Part model, mm, in its own coordinate system. A direction names the side the tool comes from. Give positions to 0.01 mm unless a question says otherwise; leave off trailing zeros. Order: outer loops, then holes, each group sorted by start corner. A loop starts at its lowest first (then second) coordinate and runs counter-clockwise, first axis right, second up. Notation, with made-up numbers: M 87,-10 L 104,-10 A27 ccw 104,24 Z; hole C -1,49 d8. An arc over 180 degrees is marked long. Write each question's results on one line, items separated by ' | '. Start each with the question number.
from build123d import *

# Parameters (mm, degrees)
SKETCH_1_W                  = 55
SKETCH_1_H                  = 160
EXTRUDE_1_DEPTH             = 3
EXTRUDE_2_DEPTH             = 35
EXTRUDE_2_DEPTH_BACK        = 195
SKETCH_2_W                  = 35
SKETCH_2_H                  = 3
EXTRUDE_3_DEPTH             = 3
EXTRUDE_3_DEPTH_BACK        = 233
SKETCH_3_W                  = 15
SKETCH_3_H                  = 3
CUT_EXTRUDE_1_DEPTH         = 3
CUT_EXTRUDE_2_DEPTH         = 3
SKETCH_6_W                  = 77
SKETCH_6_H                  = 3
CUT_EXTRUDE_3_DEPTH         = 17
SKETCH_8_R                  = 2
CUT_EXTRUDE_4_DEPTH         = 3
SKETCH_9_W                  = 13
SKETCH_9_H                  = 20
CUT_EXTRUDE_5_DEPTH         = 3
FILLET_1_R                  = 10
SKETCH_10_R                 = 2
CUT_EXTRUDE_6_DEPTH         = 10
PATTERN_LINEAR_1_COUNT      = 4
PATTERN_LINEAR_1_PITCH      = 9
PATTERN_LINEAR_1_COUNT_DIR2 = 3
PATTERN_LINEAR_1_PITCH_DIR2 = 9
SKETCH_11_R                 = 2
CUT_EXTRUDE_7_DEPTH         = 10
PATTERN_LINEAR_2_COUNT      = 5
PATTERN_LINEAR_2_PITCH      = 9
PATTERN_LINEAR_2_COUNT_DIR2 = 4
PATTERN_LINEAR_2_PITCH_DIR2 = 9


with BuildPart() as part:
    # Эскиз1 → Бобышка-Вытянуть1 (new body)
    with BuildSketch(Plane(origin=(0, 0, 0), x_dir=(1, 0, 0), z_dir=(0, 1, 0))):
        Rectangle(SKETCH_1_W, SKETCH_1_H)
    extrude(amount=EXTRUDE_1_DEPTH)

    # Эскиз2 → Бобышка-Вытянуть2 (add, two sides: drawn at the far end of the back side and taken through both)
    with BuildSketch(Plane(origin=(0, 0, -80), x_dir=(-1, 0, 0), z_dir=(0, 0, -1)).offset(-EXTRUDE_2_DEPTH_BACK)):
        with Locations((0, 1.5)):
            Rectangle(SKETCH_2_W, SKETCH_2_H)
    extrude(amount=EXTRUDE_2_DEPTH + EXTRUDE_2_DEPTH_BACK)

    # Эскиз3 → Бобышка-Вытянуть3 (add, two sides: drawn at the far end of the back side and taken through both)
    with BuildSketch(Plane(origin=(0, 0, -115), x_dir=(-1, 0, 0), z_dir=(0, 0, -1)).offset(-EXTRUDE_3_DEPTH_BACK)):
        with Locations((0, 1.5)):
            Rectangle(SKETCH_3_W, SKETCH_3_H)
    extrude(amount=EXTRUDE_3_DEPTH + EXTRUDE_3_DEPTH_BACK)

    # Эскиз4 → Вырез-Вытянуть1 (cut)
    with BuildSketch(Plane(origin=(0, 3, 0), x_dir=(1, 0, 0), z_dir=(0, 1, 0))):
        Polygon((-23.5, 80), (-23.5, 74), (-24.75, 74), (-24.75, 71.5), (-23.5, 71.5), (-23.5, 65.5), (-20.5, 65.5), (-20.5, 71.5), (-19.25, 71.5), (-19.25, 74), (-20.5, 74), (-20.5, 80), align=None)
        Polygon((-13.5, 115), (-13.5, 109), (-14.75, 109), (-14.75, 106.5), (-13.5, 106.5), (-13.5, 100.5), (-10.5, 100.5), (-10.5, 106.5), (-9.25, 106.5), (-9.25, 109), (-10.5, 109), (-10.5, 115), align=None)
        Polygon((10.5, 115), (13.5, 115), (13.5, 109), (14.75, 109), (14.75, 106.5), (13.5, 106.5), (13.5, 100.5), (10.5, 100.5), (10.5, 106.5), (9.25, 106.5), (9.25, 109), (10.5, 109), align=None)
        Polygon((20.5, 80), (23.5, 80), (23.5, 74), (24.75, 74), (24.75, 71.5), (23.5, 71.5), (23.5, 65.5), (20.5, 65.5), (20.5, 71.5), (19.25, 71.5), (19.25, 74), (20.5, 74), align=None)
        Polygon((-10.5, -115), (-13.5, -115), (-13.5, -109), (-14.75, -109), (-14.75, -106.5), (-13.5, -106.5), (-13.5, -100.5), (-10.5, -100.5), (-10.5, -106.5), (-9.25, -106.5), (-9.25, -109), (-10.5, -109), align=None)
        Polygon((13.5, -115), (13.5, -109), (14.75, -109), (14.75, -106.5), (13.5, -106.5), (13.5, -100.5), (10.5, -100.5), (10.5, -106.5), (9.25, -106.5), (9.25, -109), (10.5, -109), (10.5, -115), align=None)
        Polygon((-20.5, -80), (-23.5, -80), (-23.5, -74), (-24.75, -74), (-24.75, -71.5), (-23.5, -71.5), (-23.5, -65.5), (-20.5, -65.5), (-20.5, -71.5), (-19.25, -71.5), (-19.25, -74), (-20.5, -74), align=None)
        Polygon((23.5, -80), (23.5, -74), (24.75, -74), (24.75, -71.5), (23.5, -71.5), (23.5, -65.5), (20.5, -65.5), (20.5, -71.5), (19.25, -71.5), (19.25, -74), (20.5, -74), (20.5, -80), align=None)
    extrude(amount=-CUT_EXTRUDE_1_DEPTH, mode=Mode.SUBTRACT)

    # Эскиз5 → Вырез-Вытянуть2 (cut)
    with BuildSketch(Plane(origin=(0, 3, 0), x_dir=(1, 0, 0), z_dir=(0, 1, 0))):
        Polygon((-27.5, 51.5), (-21.5, 51.5), (-21.5, 52.75), (-19, 52.75), (-19, 51.5), (-13, 51.5), (-13, 48.5), (-19, 48.5), (-19, 47.25), (-21.5, 47.25), (-21.5, 48.5), (-27.5, 48.5), align=None)
        Polygon((-27.5, -48.5), (-27.5, -51.5), (-21.5, -51.5), (-21.5, -52.75), (-19, -52.75), (-19, -51.5), (-13, -51.5), (-13, -48.5), (-19, -48.5), (-19, -47.25), (-21.5, -47.25), (-21.5, -48.5), align=None)
    extrude(amount=-CUT_EXTRUDE_2_DEPTH, mode=Mode.SUBTRACT)

    # Эскиз6 → Вырез-Вытянуть3 (cut)
    with BuildSketch(Plane.ZY.offset(27.5)):
        with Locations((0, 1.5)):
            Rectangle(SKETCH_6_W, SKETCH_6_H)
    extrude(amount=-CUT_EXTRUDE_3_DEPTH, mode=Mode.SUBTRACT)

    # Эскиз8 → Вырез-Вытянуть4 (cut)
    with BuildSketch(Plane(origin=(0, 3, 0), x_dir=(1, 0, 0), z_dir=(0, 1, 0))):
        with Locations(Location((-13.5, -77, 0), (0, 0, 270))):
            Circle(SKETCH_8_R)
        with Locations(Location((14.5, -45, 0), (0, 0, 270))):
            Circle(SKETCH_8_R)
    extrude(amount=-CUT_EXTRUDE_4_DEPTH, mode=Mode.SUBTRACT)

    # Эскиз9 → Вырез-Вытянуть5 (cut)
    with BuildSketch(Plane(origin=(0, 3, 0), x_dir=(1, 0, 0), z_dir=(0, 1, 0))):
        with Locations((21, 0)):
            Rectangle(SKETCH_9_W, SKETCH_9_H)
    extrude(amount=-CUT_EXTRUDE_5_DEPTH, mode=Mode.SUBTRACT)

    # Скругление1
    fillet_1_edges = [part.edges().sort_by_distance(p)[0] for p in [
        (27.5, 1.5, -10),
        (27.5, 1.5, 10),
    ]]
    fillet(fillet_1_edges, radius=FILLET_1_R)

    # Эскиз10 → Вырез-Вытянуть6 (cut)
    with BuildSketch(Plane(origin=(0, 3, 0), x_dir=(1, 0, 0), z_dir=(0, 1, 0))):
        with Locations(Location((21.127265004, -35.602070686, 0), (0, 0, 270))):
            Circle(SKETCH_10_R)
    cut_extrude_6 = extrude(amount=-CUT_EXTRUDE_6_DEPTH, mode=Mode.SUBTRACT)

    # Линейный массив1: Cut-Extrude 6 4 × 3
    with Locations(*[(-i * PATTERN_LINEAR_1_PITCH, 0, -j * PATTERN_LINEAR_1_PITCH_DIR2) for i in range(PATTERN_LINEAR_1_COUNT) for j in range(PATTERN_LINEAR_1_COUNT_DIR2) if (i, j) != (0, 0)]):
        add(cut_extrude_6, mode=Mode.SUBTRACT)

    # Эскиз11 → Вырез-Вытянуть7 (cut)
    with BuildSketch(Plane(origin=(0, 3, 0), x_dir=(1, 0, 0), z_dir=(0, 1, 0))):
        with Locations(Location((21.311341687, 18.91955772, 0), (0, 0, 270))):
            Circle(SKETCH_11_R)
    cut_extrude_7 = extrude(amount=-CUT_EXTRUDE_7_DEPTH, mode=Mode.SUBTRACT)

    # Линейный массив2: Cut-Extrude 7 5 × 4
    with Locations(*[(-j * PATTERN_LINEAR_2_PITCH_DIR2, 0, -i * PATTERN_LINEAR_2_PITCH) for i in range(PATTERN_LINEAR_2_COUNT) for j in range(PATTERN_LINEAR_2_COUNT_DIR2) if (i, j) != (0, 0)]):
        add(cut_extrude_7, mode=Mode.SUBTRACT)


solid = part.part
(1) Saw through at A-A on z = 77. Give the cut face in (x, y), plus the area to 3 significant figures.
(2) Saw through at B-B on z = 45. Give the cut face in (x, y), plus the area to 3 significant figures.
(3) Probe L1, parallel to Z at x = -10, y = 0.45; L2, parallel to X at y = 0.7, z = -101; L3, parallel to Z at x = -16, y = 0.65. List the from-to ranges inside material, lowest first.
(4) Saw through at D-D on z = 3. Give the cut face in (x, y), plus the area to 3 significant figures.
(5) Tool access for faces 1 (the cylindrical face through (24.65, 1.48, -13.01)), 2 (the cylindrical face through (-5.601, 1.521, -29.918)): list every direction of +Z, -Z, +X, -X, +Y, -Y with a clear straight run to the whole face (end or side of a thin tool).
(6) Saw through at C-C on y = 2.3. Give the number of separate pieces and of enclosed holes in the cut face, plus the area to 3 significant figures.
(7) Drop flat-ended pins along their axis: P1, Ø0.6, axis at x = 14, y = 1, coming from the +Z side; P2, Ø0.6, axis at x = 10, y = 1, coming from the -Z side; P3, Ø3, axis at x = -5.69, z = -36.92, coming from the +Y side; P4, Ø1.5, axis at y = 2.5, z = 20.5, coming from the -X side. Give the stop position or say it passes through.
Taken from the geometry:
1) outline: M -27.5,0 L -23.5,0 L -23.5,3 L -27.5,3 Z; M -20.5,0 L -15.5,0 L -15.5,3 L -20.5,3 Z; M -11.5,0 L 20.5,0 L 20.5,3 L -11.5,3 Z; M 23.5,0 L 27.5,0 L 27.5,3 L 23.5,3 Z | area: 135 mm²
2) outline: M -27.5,0 L 12.5,0 L 12.5,3 L -27.5,3 Z; M 16.5,0 L 27.5,0 L 27.5,3 L 16.5,3 Z | area: 153 mm²
3) L1: z = -115 to -109, -106.5 to 106.5, 109 to 115 | L2: x = -17.5 to -13.5, -10.5 to 10.5, 13.5 to 17.5 | L3: z = -115 to -51.5, -48.5 to -38.5, 38.5 to 48.5, 51.5 to 115
4) outline: M -10.5,0 L 14.5,0 L 14.5,3 L -10.5,3 Z | area: 75.0 mm²
5) face 1: +X, +Y, -Y | face 2: +Y, -Y
6) separate pieces: 1 | enclosed holes: 34 | area: 8,800 mm²
7) P1: stops at z = 115 | P2: stops at z = -115 | P3: passes through | P4: stops at x = -10.5
